Source: CAD feature listing. Evaluate the final solid. Frame: model axes, mm. Give positions to 0.01 mm unless a question says otherwise; leave off trailing zeros. Write each loop counter-clockwise with the first axis right and the second up, starting at its lowest first coordinate (ties: lowest second). Pieces come first, ordered by that corner, then holes. Notation, with made-up numbers: M -28.5,-3 L -19.5,-3 A34 cw -19.5,34 Z; hole C -22,38 d5. An arc over 180 degrees is marked long. Return JSON: item names as keys, results as strings.
```python
from build123d import *

# Parameters (mm, degrees)
ESQUISSE1_W        = 19
ESQUISSE1_H        = 39
ESQUISSE1_R        = 3
BOSS_EXTRU_1_DEPTH = 29


with BuildPart() as part:
    # Esquisse1 → Boss.-Extru.1 (new body)
    with BuildSketch(Plane.XY):
        with Locations((9.5, 19.5)):
            Rectangle(ESQUISSE1_W, ESQUISSE1_H)
        with Locations(Location((9.5, 19.5, 0), (0, 0, 180))):
            Circle(ESQUISSE1_R, mode=Mode.SUBTRACT)
    extrude(amount=BOSS_EXTRU_1_DEPTH)


solid = part.part
```
1) Cut plane C-C, the plane z = 27. Return the cut outline in (x, y), then the cut area to 3 significant figures.
Numbers:
{"outline": "M 0,0 L 19,0 L 19,39 L 0,39 Z; hole C 9.5,19.5 d6", "area": "713 mm²"}
2) Contact query for a flat-ended pin moving along its axis: pin 1 Ø3 at (x, y) = (15.5, 26) entering from -Z. Output: stop coordinate, or through.
Numbers:
{"pin 1": "stops at z = 0"}
3) Cut plane A-A, the plane x = 9.5. Return the cut outline in (y, z), then the cut area to 3 significant figures.
Numbers:
{"outline": "M 0,0 L 16.5,0 L 16.5,29 L 0,29 Z; M 22.5,0 L 39,0 L 39,29 L 22.5,29 Z", "area": "957 mm²"}
4) Line query: line 1 (Y direction, x = 9.5, z = 6.75); line 2 (X direction, y = 19.5, z = 17.75); line 3 (X direction, y = 22, z = 4.5). Output: solid intervals per line, ascending. Write a range as [from, to].
Numbers:
{"line 1": "y = [0, 16.5], [22.5, 39]", "line 2": "x = [0, 6.5], [12.5, 19]", "line 3": "x = [0, 7.84], [11.16, 19]"}
5) Cut plane B-B, the plane y = 19.5. Return the cut outline in (x, z), then the cut area to 3 significant figures.
Numbers:
{"outline": "M 0,0 L 6.5,0 L 6.5,29 L 0,29 Z; M 12.5,0 L 19,0 L 19,29 L 12.5,29 Z", "area": "377 mm²"}
6) Draft query along Y for faces 1 (the face through (10.15, 22.43, 14.3)), 2 (the face through (5, 20, 29)), 3 (the face through (9, 0, 14)). Return one class per face: released by +Y, released by -Y, zero draft, split by the parting line, or undercut.
Numbers:
{"face 1": "undercut", "face 2": "zero draft", "face 3": "released by -Y"}
